from build123d import *

# Parameters (mm, degrees)
EXTRUDE_1_DEPTH     = 4.5
SKETCH_3_R          = 2
CUT_EXTRUDE_1_DEPTH = 10


with BuildPart() as part:
    # 草图1 → 凸台-拉伸1 (new body)
    with BuildSketch(Plane(origin=(0, 0, 0), x_dir=(1, 0, 0), z_dir=(0, 1, 0))):
        Polygon((-224.5, 274.3), (224.5, 274.3), (103, 0), (-103, 0), align=None)
    extrude(amount=EXTRUDE_1_DEPTH)

    # 草图3 → 切除-拉伸1 (cut)
    with BuildSketch(Plane(origin=(0, 4.5, 0), x_dir=(1, 0, 0), z_dir=(0, 1, 0))):
        with Locations(Location((-145, 259.3, 0), (0, 0, 270))):
            Circle(SKETCH_3_R)
        with Locations(Location((-125, 259.3, 0), (0, 0, 270))):
            Circle(SKETCH_3_R)
        with Locations(Location((125, 259.3, 0), (0, 0, 90))):
            Circle(SKETCH_3_R)
        with Locations(Location((145, 259.3, 0), (0, 0, 90))):
            Circle(SKETCH_3_R)
        with Locations(Location((-65, 10, 0), (0, 0, 270))):
            Circle(SKETCH_3_R)
        with Locations(Location((-55, 10, 0), (0, 0, 270))):
            Circle(SKETCH_3_R)
        with Locations(Location((55, 10, 0), (0, 0, 90))):
            Circle(SKETCH_3_R)
        with Locations(Location((65, 10, 0), (0, 0, 90))):
            Circle(SKETCH_3_R)
    extrude(amount=-CUT_EXTRUDE_1_DEPTH, mode=Mode.SUBTRACT)


solid = part.part
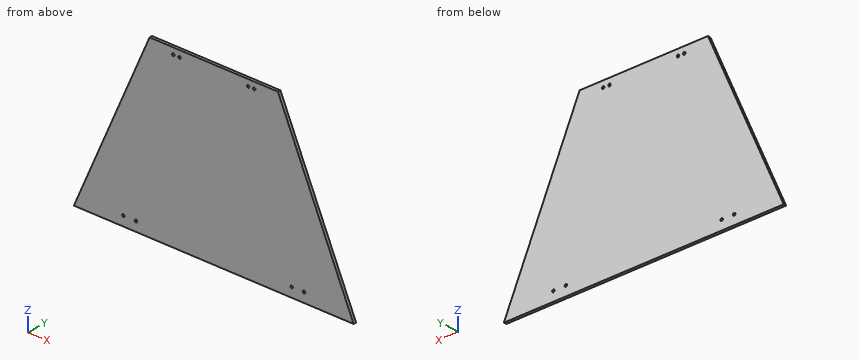
Verification items for the finished model (mm, model axes). Give positions to 0.01 mm unless a question says otherwise; leave off trailing zeros. Loops run counter-clockwise (first coordinate to the right, second up) from the corner with the lowest first, then second, coordinate; pieces in that order, holes last.
1) Thickness scan on line 1 along Z through (x, y) = (65, 1.7); line 2 along X through (y, z) = (2.15, -10); line 3 along X through (y, z) = (3.25, -259.3). Record the ranges inside material, lowest first.
2) Depth check by flat-ended pin: pin 1 Ø1.5 at (y, z) = (0.5, -62) entering from -X; pin 2 Ø3.5 at (x, z) = (-145, -259.3) entering from +Y; pin 3 Ø1.5 at (y, z) = (1, -101) entering from +X; pin 4 Ø2 at (y, z) = (3, -30) entering from -X. Enter the tip coordinate at first touch or a pass-through.
3) Sectioned sample at C-C, the plane z = -147.5. Enter the section's corners in (x, y).
4) Sectioned sample at A-A, the plane y = 2.7. Count the separate pieces of the cut face and the enclosed holes in it, then the cut area to 3 significant figures.
5) Sectioned sample at B-B, the plane x = 180.5. Enter the section's corners in (y, z).
Answers:
1. line 1: z = -274.3 to -12, -8 to 0
1. line 2: x = -107.43 to -67, -63 to -57, -53 to 53, 57 to 63, 67 to 107.43
1. line 3: x = -217.86 to -147, -143 to -127, -123 to 123, 127 to 143, 147 to 217.86
2. pin 1: stops at x = -130.79
2. pin 2: passes through
2. pin 3: stops at x = 148.07
2. pin 4: stops at x = -116.73
3. outline: (-168.33, 0) - (168.33, 0) - (168.33, 4.5) - (-168.33, 4.5) - close
4. separate pieces: 1
4. enclosed holes: 8
4. area: 89,700 mm2
5. outline: (0, -274.3) - (4.5, -274.3) - (4.5, -174.97) - (0, -174.97) - close
